```python
from build123d import *

# Parameters (mm, degrees)
SKETCH1_W                   = 25.978283713
SKETCH1_H                   = 59.69
BOSS_EXTRUDE1_DEPTH         = 7.62
SKETCH2_W                   = 25.978283713
SKETCH2_H                   = 12.7
BOSS_EXTRUDE2_DEPTH         = 12.7
SKETCH4_R                   = 14.7955
CUT_EXTRUDE1_DEPTH          = 20.32
F_1_4_CLEARANCE_HOLE1_D     = 6.7564
F_1_4_CLEARANCE_HOLE1_DEPTH = 7.62
FILLET1_R                   = 6.35
FILLET2_R                   = 2.54
F_1_4_CLEARANCE_HOLE2_D     = 6.7564


with BuildPart() as part:
    # Sketch1 → Boss-Extrude1 (new body)
    with BuildSketch(Plane(origin=(0, 0, 0), x_dir=(1, 0, 0), z_dir=(0, 1, 0))):
        with Locations((12.989141857, 29.845)):
            Rectangle(SKETCH1_W, SKETCH1_H)
    extrude(amount=BOSS_EXTRUDE1_DEPTH)

    # Sketch2 → Boss-Extrude2 (add)
    with BuildSketch(Plane(origin=(0, 7.62, 0), x_dir=(1, 0, 0), z_dir=(0, 1, 0))):
        with Locations((12.989141857, 6.35)):
            Rectangle(SKETCH2_W, SKETCH2_H)
    extrude(amount=BOSS_EXTRUDE2_DEPTH)

    # Sketch4 → Cut-Extrude1 (cut)
    with BuildSketch(Plane(origin=(0, 20.32, 0), x_dir=(1, 0, 0), z_dir=(0, 1, 0))):
        with Locations((12.989141856, -8.89)):
            Circle(SKETCH4_R)
    extrude(amount=-CUT_EXTRUDE1_DEPTH, mode=Mode.SUBTRACT)

    # 1/4 Clearance Hole1
    with Locations(Plane(origin=(0, 7.62, 0), x_dir=(1, 0, 0), z_dir=(0, 1, 0))):
        with Locations((12.989141856, 50.8), (12.989141856, 22.86)):
            Hole(F_1_4_CLEARANCE_HOLE1_D / 2, depth=F_1_4_CLEARANCE_HOLE1_DEPTH)

    # Fillet1
    fillet1_edges = [part.edges().sort_by_distance(p)[0] for p in [
        (0, 3.81, -59.69),
        (25.978283713, 3.81, -59.69),
    ]]
    fillet(fillet1_edges, radius=FILLET1_R)

    # Fillet2
    fillet2_edges = [part.edges().sort_by_distance(p)[0] for p in [
        (0, 13.97, -12.7),
        (25.978283713, 13.97, -12.7),
    ]]
    fillet(fillet2_edges, radius=FILLET2_R)

    # 1/4 Clearance Hole2 (through all)
    with Locations(Plane(origin=(0, 0, -12.7), x_dir=(-1, 0, 0), z_dir=(0, 0, -1))):
        with Locations((-12.989141856, 13.97)):
            Hole(F_1_4_CLEARANCE_HOLE2_D / 2)


solid = part.part
```
Work out the finished part from the listing and answer in its coordinate system (mm). A direction names the side the tool comes from. Coordinates: 2 decimals unless noted, no trailing zeros. Order: outer loops, then holes, each group sorted by start corner. A loop starts at its lowest first (then second) coordinate and runs counter-clockwise, first axis right, second up. Notation, with made-up numbers: M -36.5,40 L 4.5,40 A19 cw 4.5,77 Z; hole C -8.5,44 d11. An arc over 180 degrees is marked long. Use CSV: the item, a comma, the result in double quotes.
1) Section A-A on z = -22.86 is taken. Write down the section's boundary in (x, y).
Worked out:
outline,"M 0,0 L 9.61,0 L 9.61,7.62 L 0,7.62 Z; M 16.37,0 L 25.98,0 L 25.98,7.62 L 16.37,7.62 Z"
2) Determine the mould class of faces 1 (the face through (25.21, 14.06, -11.98)), 2 (the face through (1.81, 3.86, -57.78)), 3 (the face through (13.181, 10.302, -5.904)) for opening direction X: released by +X, released by -X, zero draft, split by the parting line, or undercut.
Worked out:
face 1,"released by +X"
face 2,"released by -X"
face 3,"undercut"
3) Section B-B on y = 13.97 is taken. Write down the section's boundary in (x, z), plus the area to 3 significant figures.
Worked out:
outline,"M 0,-10.16 A2.54 ccw 2.54,-12.7 L 9.61,-12.7 L 9.61,-5.51 A14.8 cw 1.16,0 L 0,0 Z; M 16.37,-12.7 L 23.44,-12.7 A2.54 ccw 25.98,-10.16 L 25.98,0 L 24.82,0 A14.8 cw 16.37,-5.51 Z"
area,"183 mm^2"
4) Section D-D on x = 22 is taken. Write down the section's boundary in (y, z).
Worked out:
outline,"M 0,-59.23 L 7.62,-59.23 L 7.62,-12.7 L 20.32,-12.7 L 20.32,-2.85 L 0,-2.85 Z"
5) For faces 4 (the face through (11, 11, -12.7)), 5 (the face through (0.724, 14.059, -11.936)), 6 (the face through (13, 0, -30)), determine the directions among +Z, -Z, +X, -X, +Y, -Y from which every point of the face is accessible in a straight line to the end or side of a thin tool.
Worked out:
face 4,"-Z, +X, -X, +Y"
face 5,"-Z, -X, +Y"
face 6,"+Z, -Z, +X, -X, -Y"
6) Consider line 1 (X direction, y = 5.75, z = -50.8); line 2 (Z direction, x = 11.5, y = 7.5); line 3 (Z direction, x = 12.75, y = 3.25). Determine where each line is inside the solid, lowest interval first. Write a range as [from, to].
Worked out:
line 1,"x = [0, 9.61], [16.37, 25.98]"
line 2,"z = [-59.69, -53.83], [-47.77, -25.89], [-19.83, -5.83]"
line 3,"z = [-59.69, -54.17], [-47.43, -26.23], [-19.49, -5.9]"
7) Section C-C on y = 6.5 is taken. Write down the section's boundary in (x, z), plus the area to 3 significant figures.
Worked out:
outline,"M 0,-53.34 A6.35 ccw 6.35,-59.69 L 19.63,-59.69 A6.35 ccw 25.98,-53.34 L 25.98,0 L 24.82,0 A14.8 cw 1.16,0 L 0,0 Z; hole C 12.99,-50.8 d6.76; hole C 12.99,-22.86 d6.76"
area,"1,360 mm^2"
8) Flat-ended cylindrical pins translate along their axes: pin 1 Ø13 at (x, z) = (13, -32) entering from +Y; pin 2 Ø4 at (x, y) = (21.5, 13.5) entering from +Z; pin 3 Ø5 at (x, y) = (7.5, 8) entering from +Z. Find the tip coordinate at first contact, or state that the pin passes through.
Worked out:
pin 1,"stops at y = 7.62"
pin 2,"stops at z = -1.52"
pin 3,"stops at z = -3.56"
